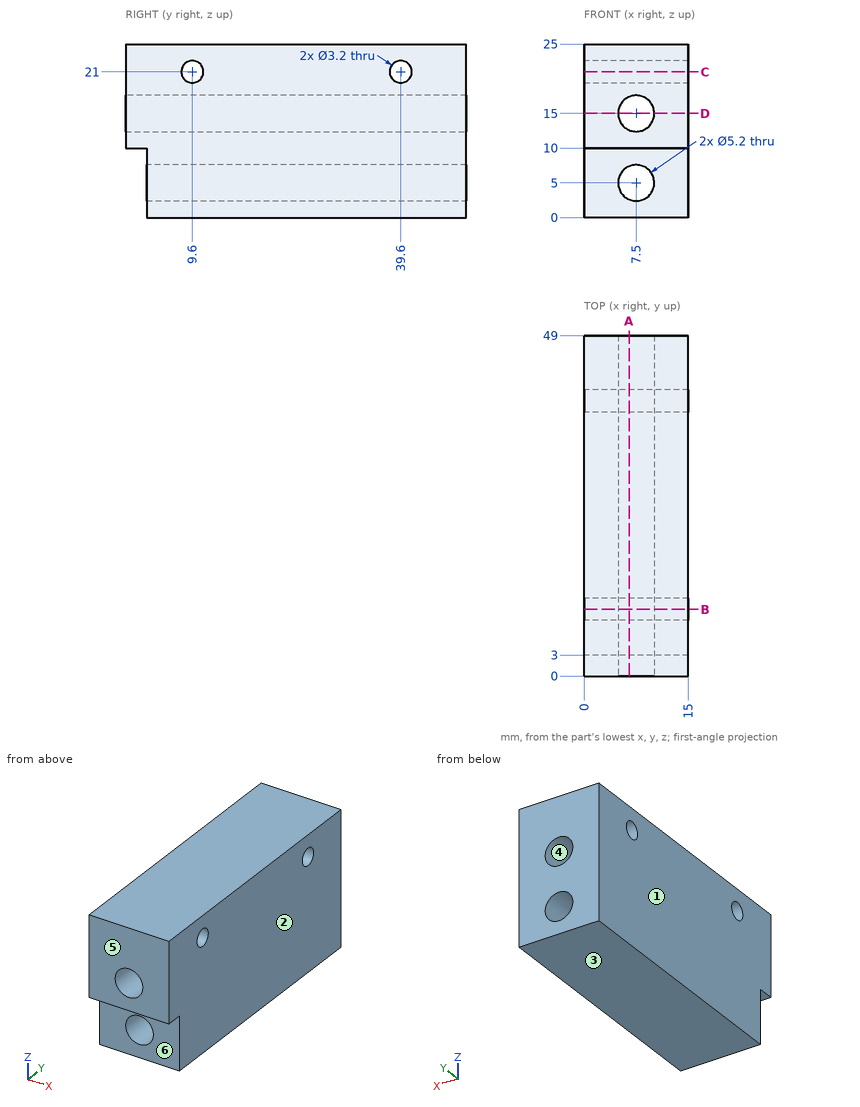
Print and shaded views of the part. All mm, measured from the part's lowest x, y and z. A direction names the side the tool comes from. Round coordinates to 2 decimals unless told otherwise and drop trailing zeros. Order: outer loops, then holes, each group sorted by start corner. A loop starts at its lowest first (then second) coordinate and runs counter-clockwise, first axis right, second up. Notation, with made-up numbers: (-22, -8.5) - (5, -8.5) arc R21 cw to (5, -1.5) - close; hole circle Ø5 at (26.5, 13.5). An arc over 180 degrees is marked (long way). Use a Markdown table: item, result.
1) Pull direction X, two halves, no side cores. Call the marked faces 1, 2, 3 and 4: pulls with the +X half, pulls with the -X half, needs draft (parallel to the pull), parting line crosses it, or undercut.
Recorded:
| item | result |
|---|---|
| face 1 | pulls with the -X half |
| face 2 | pulls with the +X half |
| face 3 | needs draft |
| face 4 | undercut |
2) Tool access for the marked faces 5 and 6: list every direction of +Z, -Z, +X, -X, +Y, -Y with a clear straight run to the whole face (end or side of a thin tool).
Recorded:
| item | result |
|---|---|
| face 5 | +Z, -Z, +X, -X, -Y |
| face 6 | -Z, +X, -X, -Y |
3) Saw through at D-D on z = 15. Write the cut outline in (x, y).
Recorded:
| item | result |
|---|---|
| outline | (0, 0) - (4.9, 0) - (4.9, 49) - (0, 49) - close; (10.1, 0) - (15, 0) - (15, 49) - (10.1, 49) - close |
4) Saw through at B-B on y = 9.6. Write the cut outline in (x, z), and give its area (3 significant figures).
Recorded:
| item | result |
|---|---|
| outline | (0, 0) - (15, 0) - (15, 19.4) - (0, 19.4) - close; (0, 22.6) - (15, 22.6) - (15, 25) - (0, 25) - close; hole circle Ø5.2 at (7.5, 5); hole circle Ø5.2 at (7.5, 15) |
| area | 285 mm² |
5) Flat gauge pin, fed straight in: pin 1 Ø1.5 at (x, y) = (5, 1.5) entering from -Z. Where does the tip first touch, or does it go through?
Recorded:
| item | result |
|---|---|
| pin 1 | stops at z = 10 |
6) Wall check: L1, parallel to Y at x = 1.25, z = 21; L2, parallel to X at y = 38.5, z = 5; L3, parallel to Z at x = 6.5, y = 13.5. Give the ranges that are in metal, low to high.
Recorded:
| item | result |
|---|---|
| L1 | y = 0 to 8, 11.2 to 38, 41.2 to 49 |
| L2 | x = 0 to 4.9, 10.1 to 15 |
| L3 | z = 0 to 2.6, 7.4 to 12.6, 17.4 to 25 |
7) Saw through at C-C on z = 21. Write the cut outline in (x, y).
Recorded:
| item | result |
|---|---|
| outline | (0, 0) - (15, 0) - (15, 8) - (0, 8) - close; (0, 11.2) - (15, 11.2) - (15, 38) - (0, 38) - close; (0, 41.2) - (15, 41.2) - (15, 49) - (0, 49) - close |
8) Saw through at A-A on x = 6.5. Write the cut outline in (y, z), and give its area (3 significant figures).
Recorded:
| item | result |
|---|---|
| outline | (0, 10) - (3, 10) - (3, 7.4) - (49, 7.4) - (49, 12.6) - (0, 12.6) - close; (0, 17.4) - (49, 17.4) - (49, 25) - (0, 25) - close; (3, 0) - (49, 0) - (49, 2.6) - (3, 2.6) - close; hole circle Ø3.2 at (9.6, 21); hole circle Ø3.2 at (39.6, 21) |
| area | 723 mm² |
